Could you check a few things on this model? Use its own coordinates, in mm. A direction names the side the tool comes from. Give positions to 0.01 mm unless a question says otherwise; leave off trailing zeros. Order: outer loops, then holes, each group sorted by start corner. A loop starts at its lowest first (then second) coordinate and runs counter-clockwise, first axis right, second up. Notation, with made-up numbers: (89.5, 2) -> (132.5, 2) arc R13 ccw to (132.5, 16) -> close; hole circle Ø7 at (-19.75, -7.5). An arc over 180 degrees is marked (long way). Answer as CSV lines item,"result". Start each with the question number.
(1) I want a section at C-C (x = -3). Please give me the cut outline in (y, z), plus the area to 3 significant figures.
(2) I want a section at D-D (y = 18.5). Please give me the cut outline in (x, z), plus the area to 3 significant figures.
(3) We'd pull the mould along Y, two halves only. Please class faces 5 (the face through (-3.3, -5.588, 4.5)), 6 (the face through (-1.875, -0.153, 4.462)), 7 (the face through (-7.608, -0.5, 4.5)): released by +Y, released by -Y, zero draft, split by the parting line, or undercut.
(4) I want a section at A-A (y = 32.5). Please give me the cut outline in (x, z).
(5) I need wall thicknesses on L1, parallel to Y at x = -4, z = 4.3; L2, parallel to Z at x = -5.25, y = 8; L3, parallel to Y at x = -1.5, z = 5.6. Which ranges of each line are inside material? Lowest first, please.
(6) I want a section at B-B (z = 6.45). Please give me the cut outline in (x, y), plus the area to 3 significant figures.
(7) Will these pins go through, and if not, where does the flat tip stop? pin 1 Ø2.5 at (x, y) = (-2.5, 10) entering from +Z; pin 2 Ø0.6 at (y, z) = (-1, 4.5) entering from -X.
(8) On a 3-axis mill with a long thin cutter (end or side, diameter ignored), from which of +Z, -Z, +X, -X, +Y, -Y can I reach the whole of each face in a straight line? I mean faces 1 (the face through (-9, 4.412, 6)), 2 (the face through (-8.458, 24, 6)), 3 (the face through (1.092, -0.5, 4.5)), 4 (the face through (-3.2, 19.21, 5.97)). Say none if no direction works.
```python
from build123d import *

# Parameters (mm, degrees)
BOSS_EXTRUDE1_DEPTH        = 3
CUT_EXTRUDE1_DEPTH         = 2.2
SKETCH3_W                  = 8.7
SKETCH3_H                  = 0.8
BOSS_EXTRUDE2_DEPTH        = 10
F_3_7_3_7_DIAMETER_HOLE1_D = 4.2
F_2_9_2_9_DIAMETER_HOLE1_D = 2.9


with BuildPart() as part:
    # Sketch1 → Boss-Extrude1 (new body)
    with BuildSketch(Plane(origin=(0, 0, 4.056081063), x_dir=(-1, 0, 0), z_dir=(0, 0, -1))):
        with BuildLine():
            Line((-1.941684048, 16.511778169), (-3.591684048, 4.411778169))
            Line((-3.591684048, 4.411778169), (10.108315952, 4.411778169))
            Line((10.108315952, 4.411778169), (8.458315952, 16.511778169))
            Line((8.458315952, 16.511778169), (8.458315952, 31.511778169))
            ThreePointArc((8.458315952, 31.511778169), (3.258315952, 36.711778169), (-1.941684048, 31.511778169))
            Line((-1.941684048, 31.511778169), (-1.941684048, 16.511778169))
        make_face()
    extrude(amount=-BOSS_EXTRUDE1_DEPTH)

    # Sketch2 → Cut-Extrude1 (cut)
    with BuildSketch(Plane.XY.offset(7.056081063)):
        with BuildLine():
            Line((1.091684048, 4.411778169), (-0.558315952, 16.511778169))
            ThreePointArc((-0.558315952, 16.511778169), (-3.258315952, 19.211778169), (-5.958315952, 16.511778169))
            Line((-5.958315952, 16.511778169), (-7.608315952, 4.411778169))
            Line((-7.608315952, 4.411778169), (1.091684048, 4.411778169))
        make_face()
    extrude(amount=-CUT_EXTRUDE1_DEPTH, mode=Mode.SUBTRACT)

    # Sketch3 → Boss-Extrude2 (add)
    with BuildSketch(Plane.XZ.offset(-4.411778169)):
        with Locations((-3.258315952, 4.456081063)):
            Rectangle(SKETCH3_W, SKETCH3_H)
    extrude(amount=BOSS_EXTRUDE2_DEPTH)

    # Ø3.7 (3.7) Diameter Hole1 (through all)
    with Locations(Plane(origin=(0, 0, 4.056081063), x_dir=(-1, 0, 0), z_dir=(0, 0, -1))):
        with Locations((3.258315952, 31.511778169)):
            Hole(F_3_7_3_7_DIAMETER_HOLE1_D / 2)

    # Ø2.9 (2.9) Diameter Hole1 (through all)
    with Locations(Plane(origin=(0, 0, 4.056081063), x_dir=(-1, 0, 0), z_dir=(0, 0, -1))):
        with Locations((3.258315952, -0.588221831)):
            Hole(F_2_9_2_9_DIAMETER_HOLE1_D / 2)


solid = part.part
```
Final values:
1,outline,"(-5.59, 4.06) -> (-2.02, 4.06) -> (-2.02, 4.86) -> (-5.59, 4.86) -> close; (0.84, 4.06) -> (29.43, 4.06) -> (29.43, 7.06) -> (19.2, 7.06) -> (19.2, 4.86) -> (0.84, 4.86) -> close; (33.6, 4.06) -> (36.71, 4.06) -> (36.71, 7.06) -> (33.6, 7.06) -> close"
1,area,"57.6 mm²"
2,outline,"(-8.46, 4.06) -> (1.94, 4.06) -> (1.94, 7.06) -> (-1.43, 7.06) -> (-1.43, 4.86) -> (-5.09, 4.86) -> (-5.09, 7.06) -> (-8.46, 7.06) -> close"
2,area,"23.2 mm²"
3,face 5,"released by -Y"
3,face 6,"undercut"
3,face 7,"zero draft"
4,outline,"(-8.36, 4.06) -> (-5.11, 4.06) -> (-5.11, 7.06) -> (-8.36, 7.06) -> close; (-1.41, 4.06) -> (1.85, 4.06) -> (1.85, 7.06) -> (-1.41, 7.06) -> close"
5,L1,"-5.59 to -1.83, 0.66 to 29.55, 33.48 to 36.66"
5,L2,"4.06 to 4.86"
5,L3,"18.56 to 30.36, 32.66 to 36.41"
6,outline,"(-10.11, 4.41) -> (-7.61, 4.41) -> (-5.96, 16.51) arc R2.7 cw to (-0.56, 16.51) -> (1.09, 4.41) -> (3.59, 4.41) -> (1.94, 16.51) -> (1.94, 31.51) arc R5.2 ccw to (-8.46, 31.51) -> (-8.46, 16.51) -> close; hole circle Ø4.2 at (-3.26, 31.51)"
6,area,"234 mm²"
7,pin 1,"z = 4.86"
7,pin 2,"x = -7.61"
8,face 1,"+Z, -Z, -X, -Y"
8,face 2,"+Z, -Z, -X, +Y"
8,face 3,"+Z, -Z, +X, -Y"
8,face 4,"+Z, -Y"
